Here's how the part is built. I have some questions about the finished solid (model axes, mm). Face numbers are marked on the shaded views. A direction names the side the tool comes from. Round coordinates to 2 decimals unless told otherwise and drop trailing zeros. Answer as CSV lines item,"result".
```python
from build123d import *

# Parameters (mm, degrees)
SKIZZE1_W                       = 10
SKIZZE1_H                       = 11
AUFSATZ_LINEAR_AUSTRAGEN1_DEPTH = 9
SKIZZE2_W                       = 1.5
SKIZZE2_H                       = 1
AUFSATZ_LINEAR_AUSTRAGEN2_DEPTH = 9
AUFSATZ_LINEAR_AUSTRAGEN3_DEPTH = 4
SKIZZE4_W                       = 5
SKIZZE4_H                       = 1.5
SCHNITT_LINEAR_AUSTRAGEN1_DEPTH = 12
AUFSATZ_LINEAR_AUSTRAGEN4_DEPTH = 2.5
SKIZZE6_W                       = 3.75
SKIZZE6_H                       = 3.75
SCHNITT_LINEAR_AUSTRAGEN2_DEPTH = 10
LINEARES_MUSTER1_COUNT          = 4
LINEARES_MUSTER1_PITCH          = 4.25
LINEARES_MUSTER1_COUNT_DIR2     = 2
LINEARES_MUSTER1_PITCH_DIR2     = 4.25
SKIZZE7_W                       = 3.5
SKIZZE7_H                       = 3.5
AUFSATZ_LINEAR_AUSTRAGEN5_DEPTH = 9
LINEARES_MUSTER2_COUNT          = 3
LINEARES_MUSTER2_PITCH          = 4.25
LINEARES_MUSTER2_COUNT_DIR2     = 2
LINEARES_MUSTER2_PITCH_DIR2     = 4.25
AUFSATZ_LINEAR_AUSTRAGEN7_DEPTH = 9
LINEARES_MUSTER4_COUNT          = 4
LINEARES_MUSTER4_PITCH          = 4.25
LINEARES_MUSTER4_COUNT_DIR2     = 2
LINEARES_MUSTER4_PITCH_DIR2     = 4.25
SCHNITT_LINEAR_AUSTRAGEN4_DEPTH = 21
LINEARES_MUSTER6_COUNT          = 4
LINEARES_MUSTER6_PITCH          = 4.25
LINEARES_MUSTER6_COUNT_DIR2     = 2
LINEARES_MUSTER6_PITCH_DIR2     = 4.25


with BuildPart() as part:
    # Skizze1 → Aufsatz-Linear austragen1 (new body, symmetric)
    with BuildSketch(Plane(origin=(0, 0, 0), x_dir=(0, 0, -1), z_dir=(1, 0, 0))):
        with Locations((0, 5.5)):
            Rectangle(SKIZZE1_W, SKIZZE1_H)
    extrude(amount=AUFSATZ_LINEAR_AUSTRAGEN1_DEPTH, both=True)

    # Skizze2 → Aufsatz-Linear austragen2 (add, symmetric)
    with BuildSketch(Plane(origin=(0, 0, 0), x_dir=(0, 0, -1), z_dir=(1, 0, 0))):
        with Locations((-5.75, 0.5)):
            Rectangle(SKIZZE2_W, SKIZZE2_H)
        with Locations((5.75, 0.5)):
            Rectangle(SKIZZE2_W, SKIZZE2_H)
    extrude(amount=AUFSATZ_LINEAR_AUSTRAGEN2_DEPTH, both=True)

    # Skizze3 → Aufsatz-Linear austragen3 (add, symmetric)
    with BuildSketch(Plane(origin=(0, 0, 0), x_dir=(0, 0, -1), z_dir=(1, 0, 0))):
        with BuildLine():
            Line((5, 11), (5.571713615, 11))
            ThreePointArc((5.571713615, 11), (5.836038655, 10.149642784), (6.535856807, 9.598979842))
            ThreePointArc((6.535856807, 9.598979842), (7.23567496, 9.048316901), (7.5, 8.197959685))
            Line((7.5, 8.197959685), (7.5, 5.197959685))
            Line((7.5, 5.197959685), (8.5, 4))
            Line((8.5, 4), (8.5, 2))
            Line((8.5, 2), (6.5, 2))
            Line((6.5, 2), (6.5, 8))
            Line((6.5, 8), (5, 8))
            Line((5, 8), (5, 11))
        make_face()
    extrude(amount=AUFSATZ_LINEAR_AUSTRAGEN3_DEPTH, both=True)

    # Skizze4 → Schnitt-Linear austragen1 (cut, through all)
    with BuildSketch(Plane.XZ):
        with Locations((0, -5.75)):
            Rectangle(SKIZZE4_W, SKIZZE4_H)
    extrude(amount=-SCHNITT_LINEAR_AUSTRAGEN1_DEPTH, mode=Mode.SUBTRACT)

    # Skizze5 → Aufsatz-Linear austragen4 (add, symmetric)
    with BuildSketch(Plane(origin=(0, 0, 0), x_dir=(0, 0, -1), z_dir=(1, 0, 0))):
        Polygon((8.123516438, 4.451012129), (8.123516438, 19.870653012), (7.136310593, 21), (6.136310593, 21), (4.623516438, 19.677608169), (4.623516438, 17.677608169), (6.123516438, 17.677608169), (6.5, 8), (6.5, 2), align=None)
    extrude(amount=AUFSATZ_LINEAR_AUSTRAGEN4_DEPTH, both=True)

    # Skizze6 → Schnitt-Linear austragen2 (cut)
    with BuildSketch(Plane.XZ):
        with Locations((-6.375, -2.125)):
            Rectangle(SKIZZE6_W, SKIZZE6_H)
    schnitt_linear_austragen2 = extrude(amount=-SCHNITT_LINEAR_AUSTRAGEN2_DEPTH, mode=Mode.SUBTRACT)

    # Lineares Muster1: Schnitt-Linear austragen2 4 × 2
    with Locations(*[(i * LINEARES_MUSTER1_PITCH, 0, j * LINEARES_MUSTER1_PITCH_DIR2) for i in range(LINEARES_MUSTER1_COUNT) for j in range(LINEARES_MUSTER1_COUNT_DIR2) if (i, j) != (0, 0)]):
        add(schnitt_linear_austragen2, mode=Mode.SUBTRACT)

    # Skizze7 → Aufsatz-Linear austragen5 (add)
    with BuildSketch(Plane(origin=(0, 11, 0), x_dir=(1, 0, 0), z_dir=(0, 1, 0))):
        with Locations((-6.375, -2.125)):
            Rectangle(SKIZZE7_W, SKIZZE7_H)
    aufsatz_linear_austragen5 = extrude(amount=AUFSATZ_LINEAR_AUSTRAGEN5_DEPTH)

    # Lineares Muster2: Aufsatz-Linear austragen5 3 × 2, 4 skipped
    with Locations(*[(i * LINEARES_MUSTER2_PITCH, 0, -j * LINEARES_MUSTER2_PITCH_DIR2) for i in range(LINEARES_MUSTER2_COUNT) for j in range(LINEARES_MUSTER2_COUNT_DIR2) if (i, j) not in ((0, 0), (0, 1), (1, 0), (1, 1), (2, 0))]):
        add(aufsatz_linear_austragen5)

    # Skizze10 → Aufsatz-Linear austragen7 (add)
    with BuildSketch(Plane(origin=(0, 11, 0), x_dir=(1, 0, 0), z_dir=(0, 1, 0))):
        Polygon((-4.625, 1.375), (-5.625, 0.375), (-7.125, 0.375), (-8.125, 1.375), (-8.125, 3.875), (-4.625, 3.875), align=None)
    aufsatz_linear_austragen7 = extrude(amount=AUFSATZ_LINEAR_AUSTRAGEN7_DEPTH)

    # Lineares Muster4: Aufsatz-Linear austragen7 4 × 2, 2 skipped
    with Locations(*[(i * LINEARES_MUSTER4_PITCH, 0, j * LINEARES_MUSTER4_PITCH_DIR2) for i in range(LINEARES_MUSTER4_COUNT) for j in range(LINEARES_MUSTER4_COUNT_DIR2) if (i, j) not in ((0, 0), (0, 1), (2, 0))]):
        add(aufsatz_linear_austragen7)

    # Skizze12 → Schnitt-Linear austragen4 (cut, through all)
    with BuildSketch(Plane(origin=(0, 20, 0), x_dir=(1, 0, 0), z_dir=(0, 1, 0))):
        Polygon((-5.875, 0.875), (-5.125, 1.625), (-5.125, 3.375), (-7.625, 3.375), (-7.625, 1.625), (-6.875, 0.875), align=None)
    schnitt_linear_austragen4 = extrude(amount=-SCHNITT_LINEAR_AUSTRAGEN4_DEPTH, mode=Mode.SUBTRACT)

    # Lineares Muster6: Schnitt-Linear austragen4 4 × 2
    with Locations(*[(i * LINEARES_MUSTER6_PITCH, 0, j * LINEARES_MUSTER6_PITCH_DIR2) for i in range(LINEARES_MUSTER6_COUNT) for j in range(LINEARES_MUSTER6_COUNT_DIR2) if (i, j) != (0, 0)]):
        add(schnitt_linear_austragen4, mode=Mode.SUBTRACT)


solid = part.part
```
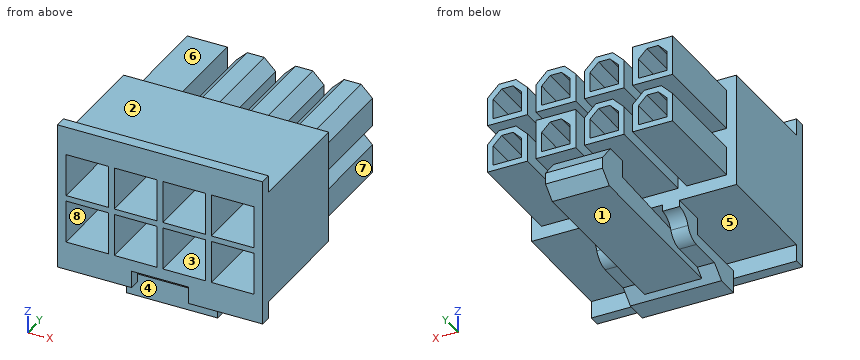
1. If we mould it in two halves opening along X, with no side actions, what happens to the marked faces 6, 7 and 8? For each: released by +X, released by -X, zero draft, split by the parting line, or undercut.
Numbers:
face 6,"zero draft"
face 7,"released by +X"
face 8,"undercut"
2. On a 3-axis mill with a long thin cutter (end or side, diameter ignored), from which of +Z, -Z, +X, -X, +Y, -Y can I reach the whole of each face in a straight line? I mean the marked faces 1, 2, 3, 4 and 5. Say none if no direction works.
Numbers:
face 1,"-Z, +X, -X, +Y"
face 2,"+Z, +X, -X, +Y"
face 3,"-Y"
face 4,"-Z, +X, -X, -Y"
face 5,"none"
3. Suppose I cut it at A-A on x = -6.5. Count the separate pieces of the cut face and the enclosed holes in it, and give its area (3 significant figures).
Numbers:
separate pieces,"3"
enclosed holes,"0"
area,"51.0 mm^2"
4. If I drill on line 1 (X direction, y = 7.5, z = -1.5); line 2 (Z direction, x = -6, y = 14) (3 decimals); line 3 (X direction, y = 10.25, z = -2.5) (3 decimals), over which ranges is the centre line in solid material (lowest first)?
Numbers:
line 1,"x = -9 to -8.25, -4.5 to -4, -0.25 to 0.25, 4 to 4.5, 8.25 to 9"
line 2,"z = -3.875 to -3.375, -0.875 to -0.375, 0.375 to 0.875, 3.375 to 3.875"
line 3,"x = -9 to -7.625, -5.125 to -3.375, -0.875 to 0.875, 3.375 to 5.125, 7.625 to 9"
5. For pin 1 Ø0.8 at (x, y) = (6.5, 16.5) entering from +Z (3 decimals); pin 2 Ø1.1 at (x, y) = (-2, 14.5) entering from -Z; pin 3 Ø3 at (x, z) = (-3, 2.5) entering from +Y, each with a flat end and sliding along its axis, tell me the tip position at first contact or that it passes through.
Numbers:
pin 1,"stops at z = 3.875"
pin 2,"stops at z = -8.12"
pin 3,"stops at y = 20"
